Geometry check sheet. Reference: the model listing, model coordinates, mm. A direction names the side the tool comes from. Coordinates: 2 decimals unless noted, no trailing zeros. Write each loop counter-clockwise with the first axis right and the second up, starting at its lowest first coordinate (ties: lowest second). Pieces come first, ordered by that corner, then holes.
from build123d import *

# Parameters (mm, degrees)
SKETCH_1_R          = 12
EXTRUDE_1_DEPTH     = 60
FILLET_1_R          = 3
SKETCH_2_W          = 4.428763437
SKETCH_2_H          = 29.827900754
CUT_EXTRUDE_1_DEPTH = 40
SKETCH_6_R          = 4
CUT_EXTRUDE_2_DEPTH = 50


with BuildPart() as part:
    # Эскиз1 → Вытянуть1 (new body)
    with BuildSketch(Plane(origin=(0, 0, 0), x_dir=(1, 0, 0), z_dir=(0, 1, 0))):
        with Locations(Location((0, 0, 0), (0, 0, 270))):
            Circle(SKETCH_1_R)
    extrude(amount=EXTRUDE_1_DEPTH)

    # Скругление1
    fillet_1_edges = [part.edges().sort_by_distance(p)[0] for p in [
        (0, 0, -12),
    ]]
    fillet(fillet_1_edges, radius=FILLET_1_R)

    # Эскиз2 → Вырез-Вытянуть1 (cut, symmetric)
    with BuildSketch(Plane.XY):
        with Locations((-11.785618281, 9.858944965)):
            Rectangle(SKETCH_2_W, SKETCH_2_H)
        with Locations((11.785618281, 9.858944965)):
            Rectangle(SKETCH_2_W, SKETCH_2_H)
    extrude(amount=CUT_EXTRUDE_1_DEPTH, both=True, mode=Mode.SUBTRACT)

    # Эскиз6 → Вырез-Вытянуть2 (cut, symmetric)
    with BuildSketch(Plane.ZY.offset(9.571236563)):
        with Locations(Location((0, 9.5, 0), (0, 0, 270))):
            Circle(SKETCH_6_R)
    extrude(amount=CUT_EXTRUDE_2_DEPTH, both=True, mode=Mode.SUBTRACT)


solid = part.part
1. Draft check along Z on faces 1 (the cylindrical face through (-0.1, 12.7, -2.4)), 2 (the flat face through (-9.571, 15, 0)), 3 (the cylindrical face through (0.53, 37.43, -11.99)). Enter one of: released by +Z, released by -Z, zero draft, split by the parting line, or undercut.
Computed values:
face 1: undercut
face 2: zero draft
face 3: split by the parting line
2. Thickness scan on line 1 along Y through (x, z) = (10, -1.5); line 2 along X through (y, z) = (12, 4.25); line 3 along Z through (x, y) = (0.75, 9.5). Record the ranges inside material, lowest first.
Computed values:
line 1: y = 24.77 to 60
line 2: x = -9.57 to 9.57
line 3: z = -11.98 to -4, 4 to 11.98
3. Sectioned sample at C-C, the plane x = 0. Record the boundary of the cut face in (y, z), and give its area (3 significant figures).
Computed values:
outline: (0, -9) arc R3 ccw to (3, -12) - (60, -12) - (60, 12) - (3, 12) arc R3 ccw to (0, 9) - close; hole circle Ø8 at (9.5, 0)
area: 1,390 mm2
4. Sectioned sample at B-B, the plane z = 0. Record the boundary of the cut face in (x, y).
Computed values:
outline: (-12, 24.77) - (-9.57, 24.77) - (-9.57, 13.5) - (9.57, 13.5) - (9.57, 24.77) - (12, 24.77) - (12, 60) - (-12, 60) - close; (-9.57, 0.05) arc R3 ccw to (-9, 0) - (9, 0) arc R3 ccw to (9.57, 0.05) - (9.57, 5.5) - (-9.57, 5.5) - close
5. Sectioned sample at D-D, the plane y = 39. Record the boundary of the cut face in (x, z), and give its area (3 significant figures).
Computed values:
outline: circle Ø24 at (0, 0)
area: 452 mm2
6. Sectioned sample at A-A, the plane y = 9.5. Record the boundary of the cut face in (x, z).
Computed values:
outline: (-9.57, -7.24) arc R12 ccw to (9.57, -7.24) - (9.57, -4) - (-9.57, -4) - close; (-9.57, 4) - (9.57, 4) - (9.57, 7.24) arc R12 ccw to (-9.57, 7.24) - close
7. Gauge pin test, flat ends, axial feed: pin 1 Ø12 at (x, y) = (-6.5, 52.5) entering from +Z; pin 2 Ø1.2 at (x, z) = (11, 2) entering from -Y; pin 3 Ø12 at (x, z) = (2.5, 4) entering from -Y; pin 4 Ø4.5 at (y, z) = (17, 0) entering from -X. Record the tip position at first contact, or that the pin passes through.
Computed values:
pin 1: stops at z = 11.99
pin 2: stops at y = 24.77
pin 3: stops at y = 0
pin 4: stops at x = -9.57
8. Access from +Z, -Z, +X, -X, +Y, -Y to the whole of each face (thin tool, end or side, straight path). Record for faces 4 (the flat face through (0, 0, 0)), 5 (the flat face through (-11, 24.773, 0)), 6 (the flat face through (9.571, 15, 0)).
Computed values:
face 4: +Z, -Z, +X, -X, -Y
face 5: +Z, -Z, -X, -Y
face 6: +Z, -Z, +X, -Y
